Source: CAD feature listing. Evaluate the final solid. Frame: model axes, mm. A direction names the side the tool comes from. Give positions to 0.01 mm unless a question says otherwise; leave off trailing zeros. Write each loop counter-clockwise with the first axis right and the second up, starting at its lowest first coordinate (ties: lowest second). Pieces come first, ordered by that corner, then holes. Notation, with made-up numbers: M -17.5,57 L -13.5,57 A23 ccw -13.5,94 Z; hole C 83.25,83.5 d3. An arc over 180 degrees is marked long. Answer as a JSON object with one key per item and string values. Group by question number.
```python
from build123d import *

# Parameters (mm, degrees)
F0_R          = 10.5
F1_DEPTH      = 4
F2_R          = 8
F3_DEPTH      = 39
F4_W          = 7
F4_H          = 5
F7_DEPTH      = 25
F7_DEPTH_BACK = 25


with BuildPart() as f1:
    # F0 (on Top) → F1 (new body)
    with BuildSketch(Plane.XY):
        Circle(F0_R)
    extrude(amount=F1_DEPTH)

    # F2 (on Top) → F3 (join)
    with BuildSketch(Plane.XY):
        Circle(F2_R)
    extrude(amount=F3_DEPTH)

    # F4 (on Right) → F5 (revolve)
    with BuildSketch(Plane.YZ):
        with Locations((3.5, 41.5)):
            Rectangle(F4_W, F4_H)
    revolve(axis=Axis((0, 0, 41.5), (0, 0, -1)))

    # F6 (on Right) → F7 (cut, two sides)
    with BuildSketch(Plane.YZ) as f7_sk:
        Polygon((0, 45), (-8, 45), (-8, 38.993425), align=None)
    extrude(amount=F7_DEPTH, mode=Mode.SUBTRACT)
    extrude(f7_sk.sketch, amount=-F7_DEPTH_BACK, mode=Mode.SUBTRACT)


solid = f1.part
```
(1) Contact query for flat-ended pins moving along their axis: pin 1 Ø3 at (x, z) = (-1, 19) entering from -Y; pin 2 Ø3 at (y, z) = (-8, 9) entering from -X; pin 3 Ø5 at (y, z) = (7, 11) entering from +X. Output: stop coordinate, or through.
(2) Access query for faces 1 (the cylindrical face through (2.103, 6.677, 41.535)), 2 (the flat face through (0, 0, 0)). Directions: +Z, -Z, +X, -X, +Y, -Y. A direction counts if a zero-diameter tool reaches every point of the face in a straight line with its end or side. Return the directions, or none.
(3) Section B-B, the plane z = 22. Return loops of the section in (x, y).
(4) Section A-A, the plane y = 0. Return loops of the section in (x, z), plus the area to 3 significant figures.
(5) Ray query, L1, parallel to Z at x = -5.5, y = -7.75; L2, parallel to Y at x = 0, z = 30. Return the intervals inside material, ascending. Write a range as [from, to].
(6) Section C-C, the plane x = -8.5. Return loops of the section in (y, z).
(7) Section D-D, the plane y = 3.5. Return loops of the section in (x, z).
Reported:
{
 "1": {"pin 1": "stops at y = -8", "pin 2": "stops at x = -4.66", "pin 3": "stops at x = 6.61"},
 "2": {"face 1": "+Z", "face 2": "-Z, +X, -X, +Y, -Y"},
 "3": {"outline": "C 0,0 d16"},
 "4": {"outline": "M -10.5,0 L 10.5,0 L 10.5,4 L 8,4 L 8,39 L 7,39 L 7,44 L -7,44 L -7,39 L -8,39 L -8,4 L -10.5,4 Z", "area": "714 mm2"},
 "5": {"L1": "z = [0, 4]", "L2": "y = [-8, 8]"},
 "6": {"outline": "M -6.16,0 L 6.16,0 L 6.16,4 L -6.16,4 Z"},
 "7": {"outline": "M -9.9,0 L 9.9,0 L 9.9,4 L 7.19,4 L 7.19,39 L 6.06,39 L 6.06,44 L -6.06,44 L -6.06,39 L -7.19,39 L -7.19,4 L -9.9,4 Z"}
}
